The drawing under review shows one solid part. Ordinate dimensions are in mm from its lowest x, y, z. Give positions to 0.01 mm unless a question says otherwise; leave off trailing zeros. Order: outer loops, then holes, each group sorted by start corner. A loop starts at its lowest first (then second) coordinate and runs counter-clockwise, first axis right, second up. Notation, with made-up numbers: (49, 43.5) - (93, 43.5) arc R25 cw to (93, 74.5) - close; hole circle Ø11 at (68, 33.5). An arc over 180 degrees is marked (long way). Write item = value, one per line. Start each with the question number.
1. Wall thickness on probe 1 along X at (y, z) = (5.9, 1.05); probe 2 along X at (y, z) = (7, 1.9); probe 3 along Y at (x, z) = (11, 0.85): over which ranges is each line inside the solid? List them lowest first.
2. We need section D-D, the plane x = 49.5. Give the boundary of the cut face in (y, z).
3. We need section A-A, the plane y = 5.9. Give the boundary of the cut face in (x, z).
4. We need section C-C, the plane z = 0.5. Give the boundary of the cut face in (x, y).
5. For P1, Ø2.5, axis at x = 56.45, y = 5.9, coming from the +Z side, flat-tipped, find the tip position at first contact; note if it passes through.
6. We need section B-B, the plane x = 56.45. Give the boundary of the cut face in (y, z).
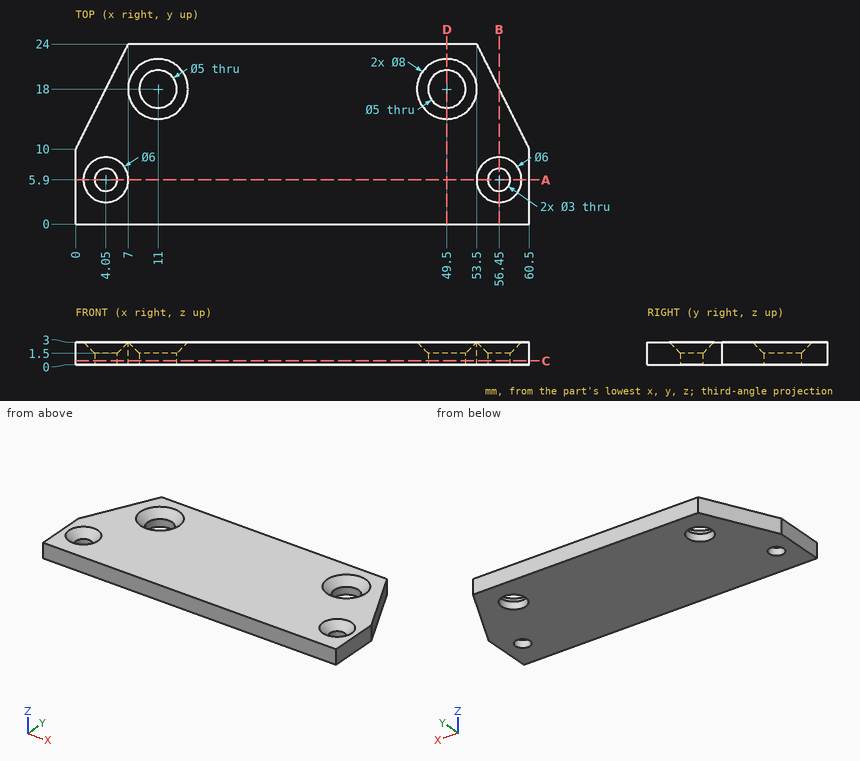
Model answer:
q1.probe_1 = 0 to 2.55, 5.55 to 54.95, 57.95 to 60.5
q1.probe_2 = 0 to 2.5, 5.6 to 54.9, 58 to 60.5
q1.probe_3 = 0 to 15.5, 20.5 to 24
q2.outline = (0, 0) - (15.5, 0) - (15.5, 1.5) - (14, 3) - (0, 3) - close; (20.5, 0) - (24, 0) - (24, 3) - (22, 3) - (20.5, 1.5) - close
q3.outline = (0, 0) - (2.55, 0) - (2.55, 1.5) - (1.05, 3) - (0, 3) - close; (5.55, 0) - (54.95, 0) - (54.95, 1.5) - (53.45, 3) - (7.05, 3) - (5.55, 1.5) - close; (57.95, 0) - (60.5, 0) - (60.5, 3) - (59.45, 3) - (57.95, 1.5) - close
q4.outline = (0, 0) - (60.5, 0) - (60.5, 10) - (53.5, 24) - (7, 24) - (0, 10) - close; hole circle Ø3 at (4.05, 5.9); hole circle Ø5 at (11, 18); hole circle Ø5 at (49.5, 18); hole circle Ø3 at (56.45, 5.9)
q5.P1 = through
q6.outline = (0, 0) - (4.4, 0) - (4.4, 1.5) - (2.9, 3) - (0, 3) - close; (7.4, 0) - (18.1, 0) - (18.1, 3) - (8.9, 3) - (7.4, 1.5) - close
